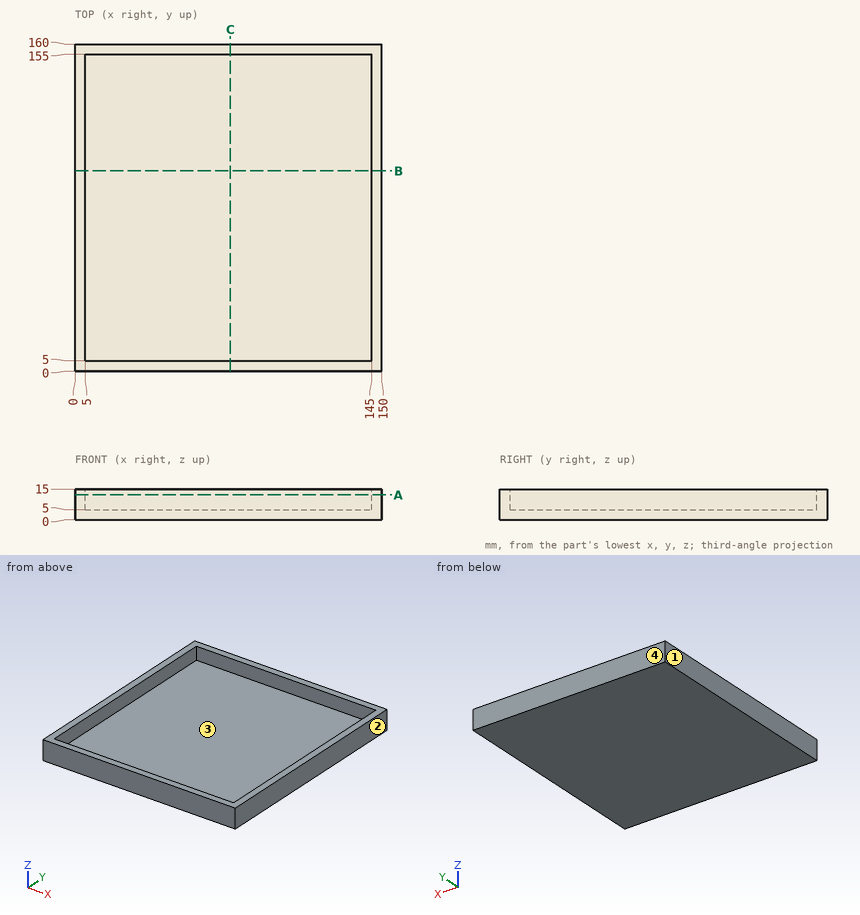
Input: dimensioned drawing with shaded views. Units: mm. Origin: part minimum x, y, z. Coordinates: 2 decimals unless noted, no trailing zeros. Loops run counter-clockwise (first coordinate to the right, second up) from the corner with the lowest first, then second, coordinate; pieces in that order, holes last.
Q1. Mould query, pull axis X, two halves, no side actions, for the marked faces 1, 2, 3 and 4. Classes: +X half, -X half, draft (parallel to the pull), parting line (faces both ways), or undercut.
Results are:
face 1: -X half
face 2: +X half
face 3: undercut
face 4: draft
Q2. Section A-A, the plane z = 12.25. Return the cut outline in (x, y).
Results are:
outline: (0, 0) - (150, 0) - (150, 160) - (0, 160) - close; hole (5, 5) - (145, 5) - (145, 155) - (5, 155) - close
Q3. Section C-C, the plane x = 76. Return the cut outline in (y, z).
Results are:
outline: (0, 0) - (160, 0) - (160, 15) - (155, 15) - (155, 5) - (5, 5) - (5, 15) - (0, 15) - close
Q4. Section B-B, the plane y = 98. Return the cut outline in (x, z).
Results are:
outline: (0, 0) - (150, 0) - (150, 15) - (145, 15) - (145, 5) - (5, 5) - (5, 15) - (0, 15) - close
Q5. Line query: line 1 along X through (y, z) = (116.5, 13); line 2 along Y through (x, z) = (7, 9.25); line 3 along Z through (x, y) = (118.5, 110). Output: solid intervals per line, ascending.
Results are:
line 1: x = 0 to 5, 145 to 150
line 2: y = 0 to 5, 155 to 160
line 3: z = 0 to 5
